Model file for the job. Use its own axes, mm. A direction names the side the tool comes from. Round coordinates to 2 decimals unless told otherwise and drop trailing zeros. Order: outer loops, then holes, each group sorted by start corner. A loop starts at its lowest first (then second) coordinate and runs counter-clockwise, first axis right, second up. Notation, with made-up numbers: (3.5, 48) -> (29.5, 48) arc R30 ccw to (29.5, 76) -> close; hole circle Ø8 at (-34, 70.25). An arc over 180 degrees is marked (long way). Put each result on its own line as item: value. Start each with the question number.
Q1. Flat gauge pins, fed straight in: P1, Ø2.5, axis at x = 18.034, z = 19.431, coming from the -Y side; P2, Ø6.5, axis at y = 14, z = 16.5, coming from the +X side; P3, Ø1.5, axis at x = 26.924, z = 0, coming from the +Y side; P4, Ø10, axis at x = 16, y = 14, coming from the +Z side. Where does each tip first touch, or does it go through?
Q2. Cut at A-A, the plane x = 0. State how many separate pieces and enclosed holes the cut face has, and give its area (3 significant figures).
Q3. Cut at D-D, the plane y = 17.5. List the corners of the cut face in (x, z) (3 decimals).
Q4. Probe L1, parallel to X at y = 12.5, z = 35; L2, parallel to Z at x = 19, y = 6 (3 decimals); L3, parallel to X at y = 1, z = 4. List the from-to ranges inside material, lowest first.
Q5. Cut at B-B, the plane z = 0. List the corners of the cut face in (x, y).
Q6. Pull direction X, two halves, no side cores. Call faces 6 (the face through (-1.904, 10.689, 37.484)), 7 (the face through (0, 10.414, 16)), 8 (the face through (2.219, 29.492, 13.705)): released by +X, released by -X, zero draft, split by the parting line, or undercut.
Q7. Cut at C-C, the plane x = 13.5. List the corners of the cut face in (y, z) (3 decimals), and give its area (3 significant figures).
Q8. 3-axis set-ups, long thin cutter, end or side, ignore diameter. For faces 1 (the face through (25.146, 12, 0)), 2 (the face through (8.51, 2.06, -5.734)), 3 (the face through (1.778, 10, 32)), 4 (the face through (13, 16, 22.225)), 5 (the face through (13, 4.064, 16)): which of +Z, -Z, +X, -X, +Y, -Y reach the whole face in a straight line?
from build123d import *

# Parameters (mm, degrees)
SKETCH1_R           = 1.25
BOSS_EXTRUDE1_DEPTH = 4.064
FILLET1_R           = 2.54
SKETCH1_5_W         = 4.064
SKETCH1_5_H         = 12.7
SKETCH1_5_R         = 1.25
SKETCH1_5_H_2       = 2.921
BOSS_EXTRUDE2_DEPTH = 21.082
SKETCH1_7_W         = 4.064
SKETCH1_7_H         = 2.921
SKETCH1_7_W_2       = 23.368
SKETCH1_7_H_2       = 12.7
BOSS_EXTRUDE3_DEPTH = 31.496
SKETCH1_9_W         = 23.368
SKETCH1_9_H         = 12.7
SKETCH1_9_W_2       = 4.064
CUT_EXTRUDE1_DEPTH  = 27.432
SKETCH1_10_W        = 23.368
SKETCH1_10_H        = 12.7
SKETCH1_10_W_2      = 4.064
BOSS_EXTRUDE4_DEPTH = 4.064
SKETCH2_R           = 1.25
CUT_EXTRUDE2_DEPTH  = 12.7
SKETCH2_3_W         = 12.7
SKETCH2_3_H         = 6.35
CUT_EXTRUDE3_DEPTH  = 40.132
FILLET2_R           = 3.81
FILLET3_R           = 1.27
SKETCH3_R           = 1.5
CUT_EXTRUDE4_DEPTH  = 19.304
FILLET4_R           = 2.286


with BuildPart() as part:
    # Sketch1 → Boss-Extrude1 (new body)
    with BuildSketch(Plane(origin=(0, 0, 0), x_dir=(1, 0, 0), z_dir=(0, 1, 0))):
        Polygon((29.21, 6.096), (8.128, 6.096), (8.128, -6.604), (1.778, -6.604), (1.778, 6.096), (-2.286, 6.096), (-2.286, -37.846), (1.778, -37.846), (1.778, -25.146), (8.128, -25.146), (8.128, -37.846), (29.21, -37.846), align=None)
        with Locations(Location((26.924, 0, 0), (0, 0, 270))):
            Circle(SKETCH1_R, mode=Mode.SUBTRACT)
        with Locations(Location((0, 0, 0), (0, 0, 270))):
            Circle(SKETCH1_R, mode=Mode.SUBTRACT)
        with Locations(Location((26.924, -31.75, 0), (0, 0, 270))):
            Circle(SKETCH1_R, mode=Mode.SUBTRACT)
        with Locations(Location((0, -31.75, 0), (0, 0, 270))):
            Circle(SKETCH1_R, mode=Mode.SUBTRACT)
    extrude(amount=BOSS_EXTRUDE1_DEPTH)

    # Fillet1
    fillet1_edges = [part.edges().sort_by_distance(p)[0] for p in [
        (8.128, 2.032, 25.146),
        (1.778, 2.032, 25.146),
        (1.778, 2.032, 6.604),
        (8.128, 2.032, 6.604),
    ]]
    fillet(fillet1_edges, radius=FILLET1_R)

    # Sketch1<5> → Boss-Extrude2 (add)
    # profile 1 of 9: a face of its own
    with BuildSketch(Plane(origin=(0, 0, 0), x_dir=(1, 0, 0), z_dir=(0, 1, 0))):
        Polygon((1.778, -22.225), (1.778, -9.525), (1.778, -6.604), (-2.286, -6.604), (-2.286, -25.146), (1.778, -25.146), align=None)
    # profile 2 of 9: a face of its own
    with BuildSketch(Plane(origin=(0, 0, 0), x_dir=(1, 0, 0), z_dir=(0, 1, 0))):
        with Locations((-0.254, -31.496)):
            Rectangle(SKETCH1_5_W, SKETCH1_5_H)
        with Locations(Location((0, -31.75, 0), (0, 0, 270))):
            Circle(SKETCH1_5_R, mode=Mode.SUBTRACT)
    # profile 3 of 9: a face of its own
    with BuildSketch(Plane(origin=(0, 0, 0), x_dir=(1, 0, 0), z_dir=(0, 1, 0))):
        with Locations((-0.254, -0.254)):
            Rectangle(SKETCH1_5_W, SKETCH1_5_H)
        with Locations(Location((0, 0, 0), (0, 0, 270))):
            Circle(SKETCH1_5_R, mode=Mode.SUBTRACT)
    # profile 4 of 9: a face of its own
    with BuildSketch(Plane(origin=(0, 0, 0), x_dir=(1, 0, 0), z_dir=(0, 1, 0))):
        Polygon((25.146, -25.146), (25.146, -22.225), (1.778, -22.225), (1.778, -25.146), (8.128, -25.146), align=None)
    # profile 5 of 9: a face of its own
    with BuildSketch(Plane(origin=(0, 0, 0), x_dir=(1, 0, 0), z_dir=(0, 1, 0))):
        Polygon((25.146, -9.525), (25.146, -6.604), (8.128, -6.604), (1.778, -6.604), (1.778, -9.525), align=None)
    # profile 6 of 9: a face of its own
    with BuildSketch(Plane(origin=(0, 0, 0), x_dir=(1, 0, 0), z_dir=(0, 1, 0))):
        with Locations((27.178, -8.0645)):
            Rectangle(SKETCH1_5_W, SKETCH1_5_H_2)
    # profile 7 of 9: a face of its own
    with BuildSketch(Plane(origin=(0, 0, 0), x_dir=(1, 0, 0), z_dir=(0, 1, 0))):
        with Locations((27.178, -23.6855)):
            Rectangle(SKETCH1_5_W, SKETCH1_5_H_2)
    # profile 8 of 9: a face of its own
    with BuildSketch(Plane(origin=(0, 0, 0), x_dir=(1, 0, 0), z_dir=(0, 1, 0))):
        with Locations((27.178, -31.496)):
            Rectangle(SKETCH1_5_W, SKETCH1_5_H)
        with Locations(Location((26.924, -31.75, 0), (0, 0, 270))):
            Circle(SKETCH1_5_R, mode=Mode.SUBTRACT)
    # profile 9 of 9: a face of its own
    with BuildSketch(Plane(origin=(0, 0, 0), x_dir=(1, 0, 0), z_dir=(0, 1, 0))):
        with Locations((27.178, -0.254)):
            Rectangle(SKETCH1_5_W, SKETCH1_5_H)
        with Locations(Location((26.924, 0, 0), (0, 0, 270))):
            Circle(SKETCH1_5_R, mode=Mode.SUBTRACT)
    extrude(amount=BOSS_EXTRUDE2_DEPTH)

    # Sketch1<7> → Boss-Extrude3 (add)
    with BuildSketch(Plane(origin=(0, 0, 0), x_dir=(1, 0, 0), z_dir=(0, 1, 0))):
        with Locations((27.178, -8.0645)):
            Rectangle(SKETCH1_7_W, SKETCH1_7_H)
        Polygon((25.146, -9.525), (25.146, -6.604), (8.128, -6.604), (1.778, -6.604), (1.778, -9.525), align=None)
        with Locations((27.178, -23.6855)):
            Rectangle(SKETCH1_7_W, SKETCH1_7_H)
        with Locations((13.462, -15.875)):
            Rectangle(SKETCH1_7_W_2, SKETCH1_7_H_2)
        with Locations((27.178, -15.875)):
            Rectangle(SKETCH1_7_W, SKETCH1_7_H_2)
        Polygon((25.146, -25.146), (25.146, -22.225), (1.778, -22.225), (1.778, -25.146), (8.128, -25.146), align=None)
        Polygon((1.778, -22.225), (1.778, -9.525), (1.778, -6.604), (-2.286, -6.604), (-2.286, -25.146), (1.778, -25.146), align=None)
    extrude(amount=BOSS_EXTRUDE3_DEPTH)

    # Sketch1<9> → Cut-Extrude1 (cut)
    with BuildSketch(Plane(origin=(0, 0, 0), x_dir=(1, 0, 0), z_dir=(0, 1, 0))):
        with Locations((13.462, -15.875)):
            Rectangle(SKETCH1_9_W, SKETCH1_9_H)
        with Locations((27.178, -15.875)):
            Rectangle(SKETCH1_9_W_2, SKETCH1_9_H)
    extrude(amount=CUT_EXTRUDE1_DEPTH, mode=Mode.SUBTRACT)

    # Sketch1<10> → Boss-Extrude4 (add)
    with BuildSketch(Plane(origin=(0, 0, 0), x_dir=(1, 0, 0), z_dir=(0, 1, 0))):
        with Locations((13.462, -15.875)):
            Rectangle(SKETCH1_10_W, SKETCH1_10_H)
        with Locations((27.178, -15.875)):
            Rectangle(SKETCH1_10_W_2, SKETCH1_10_H)
    extrude(amount=BOSS_EXTRUDE4_DEPTH)

    # Sketch2 → Cut-Extrude2 (cut)
    with BuildSketch(Plane(origin=(29.21, 0, 0), x_dir=(0, 0, -1), z_dir=(1, 0, 0))):
        with Locations((-15.875, 29.21)):
            Circle(SKETCH2_R)
        with Locations((-15.875, 2.286)):
            Circle(SKETCH2_R)
    extrude(amount=-CUT_EXTRUDE2_DEPTH, mode=Mode.SUBTRACT)

    # Sketch2<3> → Cut-Extrude3 (cut)
    with BuildSketch(Plane(origin=(29.21, 0, 0), x_dir=(0, 0, -1), z_dir=(1, 0, 0))):
        with Locations((-15.875, 24.257)):
            Rectangle(SKETCH2_3_W, SKETCH2_3_H)
        with Locations((-15.875, 7.239)):
            Rectangle(SKETCH2_3_W, SKETCH2_3_H)
    extrude(amount=-CUT_EXTRUDE3_DEPTH, mode=Mode.SUBTRACT)

    # Fillet2
    fillet2_edges = [part.edges().sort_by_distance(p)[0] for p in [
        (-0.254, 21.082, 9.525),
        (-0.254, 21.082, 22.225),
        (-0.254, 10.414, 22.225),
        (-0.254, 10.414, 9.525),
    ]]
    fillet(fillet2_edges, radius=FILLET2_R)

    # Fillet3
    fillet3_edges = [part.edges().sort_by_distance(p)[0] for p in [
        (29.21, 10.541, 37.846),
        (8.128, 2.032, 37.846),
        (-2.286, 10.541, 37.846),
        (-2.286, 10.541, -6.096),
        (8.128, 2.032, -6.096),
        (29.21, 10.541, -6.096),
    ]]
    fillet(fillet3_edges, radius=FILLET3_R)

    # Sketch3 → Cut-Extrude4 (cut)
    with BuildSketch(Plane(origin=(0, 31.496, 0), x_dir=(1, 0, 0), z_dir=(0, 1, 0))):
        with Locations(Location((2.794, -12.319, 0), (0, 0, 270))):
            Circle(SKETCH3_R)
        with Locations(Location((18.034, -12.319, 0), (0, 0, 270))):
            Circle(SKETCH3_R)
        with Locations(Location((2.794, -19.431, 0), (0, 0, 270))):
            Circle(SKETCH3_R)
        with Locations(Location((18.034, -19.431, 0), (0, 0, 270))):
            Circle(SKETCH3_R)
    extrude(amount=-CUT_EXTRUDE4_DEPTH, mode=Mode.SUBTRACT)

    # Fillet4
    fillet4_edges = [part.edges().sort_by_distance(p)[0] for p in [
        (13.462, 31.496, 6.604),
        (13.462, 31.496, 25.146),
    ]]
    fillet(fillet4_edges, radius=FILLET4_R)


solid = part.part
Ans:
1. P1: stops at y = 0
1. P2: stops at x = 1.78
1. P3: passes through
1. P4: stops at z = 25.15
2. separate pieces: 3
2. enclosed holes: 2
2. area: 863 mm^2
3. outline: (-2.286, -4.826) arc R1.27 ccw to (-1.016, -6.096) -> (1.778, -6.096) -> (1.778, 6.604) -> (25.146, 6.604) -> (25.146, -6.096) -> (27.94, -6.096) arc R1.27 ccw to (29.21, -4.826) -> (29.21, 9.525) -> (1.778, 9.525) -> (1.778, 11.215) arc R1.5 cw to (1.778, 13.423) -> (1.778, 18.327) arc R1.5 cw to (1.778, 20.535) -> (1.778, 22.225) -> (29.21, 22.225) -> (29.21, 36.576) arc R1.27 ccw to (27.94, 37.846) -> (25.146, 37.846) -> (25.146, 25.146) -> (1.778, 25.146) -> (1.778, 37.846) -> (-1.016, 37.846) arc R1.27 ccw to (-2.286, 36.576) -> close; hole circle Ø2.5 at (0, 0); hole circle Ø2.5 at (0, 31.75); hole circle Ø2.5 at (26.924, 0); hole circle Ø2.5 at (26.924, 31.75)
4. L1: x = -2.29 to 1.78, 25.15 to 29.21
4. L2: z = 6.604 to 9.525, 22.225 to 25.146
4. L3: x = -2.29 to 1.78, 8.13 to 29.21
5. outline: (-2.29, 0) -> (-1.25, 0) -> (-1.25, 21.08) -> (-2.29, 21.08) -> close; (1.25, 0) -> (1.78, 0) -> (1.78, 21.08) -> (1.25, 21.08) -> close; (8.13, 0) -> (25.67, 0) -> (25.67, 21.08) -> (25.15, 21.08) -> (25.15, 4.06) -> (8.13, 4.06) -> close; (28.17, 0) -> (29.21, 0) -> (29.21, 21.08) -> (28.17, 21.08) -> close
6. face 6: released by -X
6. face 7: zero draft
6. face 8: undercut
7. outline: (0, -6.096) -> (4.064, -6.096) -> (4.064, 6.604) -> (29.21, 6.604) arc R2.286 ccw to (31.496, 8.89) -> (31.496, 22.86) arc R2.286 ccw to (29.21, 25.146) -> (4.064, 25.146) -> (4.064, 37.846) -> (0, 37.846) -> close; hole (4.064, 9.525) -> (27.432, 9.525) -> (27.432, 22.225) -> (4.064, 22.225) -> close
7. area: 388 mm^2
8. face 1: -Z, +Y
8. face 2: -Z, +Y, -Y
8. face 3: +Z, +Y
8. face 4: +X
8. face 5: +X, -X
